Autodesk Inventor part; units mm, degrees
ref_plane "YZ Plane" through (0, 0, 0) normal (1, 0, 0) x (0, 1, 0)
ref_plane "XZ Plane" through (0, 0, 0) normal (0, 1, 0) x (-1, 0, 0)
ref_plane "XY Plane" through (0, 0, 0) normal (0, 0, 1) x (1, 0, 0)
sketch "Szkic1" plane through (0, 0, 0) normal (0, 0, 1) x (1, 0, 0)
  line L0 (-27.5, 10.1009) -> (-10, 10.1009)
  line L1 (-10, 10.1009) -> (-10, 0.1009)
  line L2 (-10, 0.1009) -> (10, 0.1009)
  line L3 (-27.5, 10.1009) -> (-27.5, -19.8991)
  line L4 (-27.5, -19.8991) -> (-15.5, -19.8991)
  line L5 (-15.5, -19.8991) -> (-15.5, -29.8991)
  line L6 (-15.5, -29.8991) -> (15.5, -29.8991)
  line L7 (27.5, 10.1009) -> (10, 10.1009)
  line L8 (10, 10.1009) -> (10, 0.1009)
  line L9 (27.5, 10.1009) -> (27.5, -19.8991)
  line L10 (27.5, -19.8991) -> (15.5, -19.8991)
  line L11 (15.5, -19.8991) -> (15.5, -29.8991)
  point P0 (0, 0)
  dimension "d1" = 55
  dimension "d2" = 17.5
  dimension "d3" = 20
  dimension "d4" = 12
  dimension "d5" = 12
  dimension "d6" = 10
  dimension "d14" = 40
  dimension "d15" = 40
  dimension "d16" = 10
  dimension "d17" = 10
extrude "Wyciągnięcie proste1" add sketch "Szkic1" along normal blind 90
sketch "Szkic3" plane through (-27.5, -19.8991, 0) normal (-1, 0, 0) x (0, 0, 1)
  line L0 (5, 30) -> (85, 30)
  line L1 (85, 30) -> (85, 20)
  line L2 (85, 20) -> (5, 20)
  line L3 (5, 20) -> (5, 30)
  line L4 (0, 30) -> (0, 0)
  line L5 (0, 30) -> (90, 30)
  point P0 (0, 19.8991)
  dimension "d19" = 5
  dimension "d20" = 10
extrude "Wyciągnięcie proste3" cut sketch "Szkic3" against normal through all
sketch "Szkic4" plane through (-15.5, -29.8991, 0) normal (-1, 0, 0) x (0, 0, 1)
  line L0 (20, 0) -> (70, 0)
  line L1 (70, 0) -> (70, 10)
  line L2 (70, 10) -> (20, 10)
  line L3 (20, 10) -> (20, 0)
  line L4 (0, 10) -> (0, 0)
  point P0 (0, 29.8991)
  dimension "d23" = 20
  dimension "d24" = 50
extrude "Wyciągnięcie proste4" cut sketch "Szkic4" against normal through all
sketch "Szkic5" plane through (-10, 0.1009, 0) normal (0, 1, 0) x (1, 0, 0)
  line L0 (0, -85) -> (0, -90) construction
  line L1 (20, -90) -> (0, -90) construction
  line L2 (20, -85) -> (20, -90) construction
  line L3 (20, -85) -> (37.5, -85) construction
  line L4 (37.5, -5) -> (37.5, -85) construction
  line L5 (20, -5) -> (37.5, -5) construction
  line L6 (20, 0) -> (20, -5) construction
  line L7 (20, 0) -> (0, 0) construction
  line L8 (0, 0) -> (0, -5) construction
  line L9 (-17.5, -5) -> (0, -5) construction
  line L10 (-17.5, -85) -> (-17.5, -5) construction
  line L11 (-17.5, -85) -> (0, -85) construction
  circle A0 centre (10, -45) radius 7.5
  point P0 (10, 0)
  dimension "d27" = 15
extrude "Wyciągnięcie proste5" cut sketch "Szkic5" against normal through all
ref_plane "Płaszczyzna konstrukcyjna1" through (0, -19.8991, 0) normal (-1, 0, 0) x (0, 0, 1)
sketch "Szkic6" plane through (0, -19.8991, 0) normal (-1, 0, 0) x (0, 0, 1)
  line L0 (85, 30) -> (85, 20)
  line L1 (85, 20) -> (5, 20)
  line L2 (5, 20) -> (5, 30)
  line L3 (0, 30) -> (5, 30)
  line L4 (0, 30) -> (0, 0)
  line L5 (0, 0) -> (90, 0)
  line L6 (90, 30) -> (90, 0)
  line L7 (85, 30) -> (90, 30)
  line L8 (70, 0) -> (20, 0)
  line L9 (20, 0) -> (20, 10)
  line L10 (20, 10) -> (70, 10)
  line L11 (70, 10) -> (70, 0)
  point P0 (0, 19.8991)
extrude "Wyciągnięcie proste6" cut sketch "Szkic6" along normal mid plane 35 contours L5 L9 L10 L11
properties part number "Bartosz_Zukowski_model_nr_5_1"
For this review, take the finished solid that the model builds, in its own axes (mm). A direction names the side the tool comes from. Coordinates: 2 decimals unless noted, no trailing zeros. Loops run counter-clockwise (first coordinate to the right, second up) from the corner with the lowest first, then second, coordinate; pieces in that order, holes last. Notation, with made-up numbers: (-24, 49) -> (30, 49) arc R21 ccw to (30, 71) -> close; hole circle Ø7 at (20.5, 16). An arc over 180 degrees is marked (long way). Write each question's results on one line, items separated by ' | '.
Q1. For pin 1 Ø4 at (x, z) = (19.5, 20) entering from -Y; pin 2 Ø13.5 at (x, z) = (0, 45) entering from +Y; pin 3 Ø10.5 at (x, z) = (4.5, 55) entering from -Y; pin 4 Ø3 at (y, z) = (-27, 75.5) entering from +X, all flat-tipped, find the tip position at first contact; note any pin that passes through.
Taken from the geometry:
pin 1: y = -19.9 | pin 2: through | pin 3: y = -9.9 | pin 4: x = 15.5
Q2. Machinability: for faces 1 (the flat face through (-15.5, -25, 80)), 2 (the flat face through (-10, 5, 2)), 3 (the flat face through (19, 5, 5)), 4 (the flat face through (0, -20, 70)), which of the approach directions +Z, -Z, +X, -X, +Y, -Y give a long, thin tool a straight path to every point of the face, cutting with its end or side? Answer none if there is none.
Taken from the geometry:
face 1: +Z, -Z, -X, -Y | face 2: +Z, -Z, +Y | face 3: +X, -X, +Y | face 4: -Y
Q3. To check wall thickness, follow line 1 along X through (y, z) = (-15, 31); line 2 along Z through (x, y) = (0, -3.25); line 3 along X through (y, z) = (-3, 45). State the ranges of each line that lie inside material, in increasing order. Write a range as [from, to].
Taken from the geometry:
line 1: [-27.5, -17.5], [17.5, 27.5] | line 2: [0, 37.5], [52.5, 90] | line 3: [-27.5, -7.5], [7.5, 27.5]
Q4. Add section C-C, the plane z = 45. State the section outline as (x, y) points.
Taken from the geometry:
outline: (-27.5, -19.9) -> (-17.5, -19.9) -> (-17.5, -9.9) -> (-7.5, -9.9) -> (-7.5, 0.1) -> (-27.5, 0.1) -> close; (7.5, -9.9) -> (17.5, -9.9) -> (17.5, -19.9) -> (27.5, -19.9) -> (27.5, 0.1) -> (7.5, 0.1) -> close
Q5. Add section D-D, the plane y = -17. State the section outline as (x, z) points, then the cut area to 3 significant figures.
Taken from the geometry:
outline: (-27.5, 0) -> (27.5, 0) -> (27.5, 90) -> (-27.5, 90) -> close; hole (-17.5, 20) -> (17.5, 20) -> (17.5, 70) -> (-17.5, 70) -> close | area: 3,200 mm²
Q6. Mouldability with a two-part tool opening along Z and no side actions: class faces 5 (the flat face through (0, 0.101, 54)), 6 (the flat face through (-27.5, -8, 44)) as +Z half, -Z half, draft (parallel to the pull), parting line (faces both ways), or undercut.
Taken from the geometry:
face 5: undercut | face 6: draft
Q7. Add section B-B, the plane y = -24.5. State the section outline as (x, z) points, then the cut area to 3 significant figures.
Taken from the geometry:
outline: (-15.5, 0) -> (15.5, 0) -> (15.5, 20) -> (-15.5, 20) -> close; (-15.5, 70) -> (15.5, 70) -> (15.5, 90) -> (-15.5, 90) -> close | area: 1,240 mm²
Q8. Add section A-A, the plane x = 0. State the section outline as (y, z) points, then the cut area to 3 significant figures.
Taken from the geometry:
outline: (-29.9, 0) -> (0.1, 0) -> (0.1, 37.5) -> (-9.9, 37.5) -> (-9.9, 20) -> (-29.9, 20) -> close; (-29.9, 70) -> (-9.9, 70) -> (-9.9, 52.5) -> (0.1, 52.5) -> (0.1, 90) -> (-29.9, 90) -> close | area: 1,550 mm²
